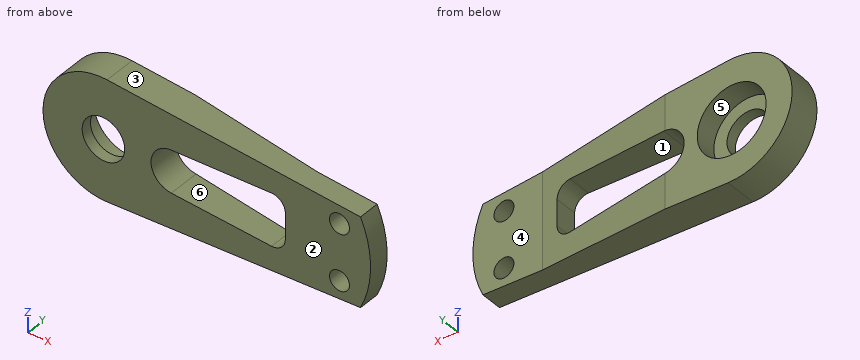
```python
from build123d import *

# Parameters (mm, degrees)
SKETCH1_R               = 1.9
SKETCH1_R_2             = 4.05
BOSS_EXTRUDE2_DEPTH     = 6
SKETCH2_R               = 6.55
CUT_EXTRUDE3_DEPTH      = 4
CUT_EXTRUDE2_DEPTH      = 21
CUT_EXTRUDE2_DEPTH_BACK = 16


with BuildPart() as part:
    # Sketch1 → Boss-Extrude2 (new body)
    with BuildSketch(Plane(origin=(0, 0, 0), x_dir=(1, 0, 0), z_dir=(0, 1, 0))):
        with BuildLine():
            Line((0.702058205, 11.478550182), (48.9, 8.530637776))
            ThreePointArc((48.9, 8.530637776), (50.810549507, 0), (48.9, -8.530637776))
            Line((48.9, -8.530637776), (0.702058205, -11.478550182))
            ThreePointArc((0.702058205, -11.478550182), (-11.5, 0), (0.702058205, 11.478550182))
        make_face()
        with Locations(Location((44.9, -5.35, 0), (0, 0, 270))):
            Circle(SKETCH1_R, mode=Mode.SUBTRACT)
        with Locations(Location((0, 0, 0), (0, 0, 270))):
            Circle(SKETCH1_R_2, mode=Mode.SUBTRACT)
        with Locations(Location((44.9, 5.35, 0), (0, 0, 270))):
            Circle(SKETCH1_R, mode=Mode.SUBTRACT)
        with BuildLine():
            Line((12.898162181, 4.044967428), (31.975408753, 4.996893474))
            ThreePointArc((31.975408753, 4.996893474), (33.823154358, 4.311281054), (34.6, 2.5))
            Line((34.6, 2.5), (34.6, -2.5))
            ThreePointArc((34.6, -2.5), (33.823154358, -4.311281054), (31.975408753, -4.996893474))
            Line((31.975408753, -4.996893474), (12.898162181, -4.044967428))
            ThreePointArc((12.898162181, -4.044967428), (9.05, 0), (12.898162181, 4.044967428))
        make_face(mode=Mode.SUBTRACT)
    extrude(amount=BOSS_EXTRUDE2_DEPTH)

    # Sketch2 → Cut-Extrude3 (cut)
    with BuildSketch(Plane(origin=(0, 6, 0), x_dir=(1, 0, 0), z_dir=(0, 1, 0))):
        with Locations(Location((0, 0, 0), (0, 0, 270))):
            Circle(SKETCH2_R)
    extrude(amount=-CUT_EXTRUDE3_DEPTH, mode=Mode.SUBTRACT)

    # Sketch3 → Cut-Extrude2 (cut, two sides: drawn at the far end of the back side and taken through both)
    with BuildSketch(Plane.XY.offset(-CUT_EXTRUDE2_DEPTH_BACK)):
        Polygon((50.810549507, 4), (37.603420494, 4), (12.707964704, 6), (50.810549507, 6), align=None)
    extrude(amount=CUT_EXTRUDE2_DEPTH + CUT_EXTRUDE2_DEPTH_BACK, mode=Mode.SUBTRACT)


solid = part.part
```
Can you work these out from the model? Positions are in its coordinate system, mm. Face numbers are marked on the shaded views. A direction names the side the tool comes from. Give positions to 0.01 mm unless a question says otherwise; leave off trailing zeros. Loops run counter-clockwise (first coordinate to the right, second up) from the corner with the lowest first, then second, coordinate; pieces in that order, holes last. Notation, with made-up numbers: M -15.75,-21.75 L 15.25,-21.75 A25 ccw 15.25,14.25 Z; hole C -23,75 d3. An arc over 180 degrees is marked long. One line per question, with ' | ' between items. Start each with the question number.
Q1. If we section it at C-C (y = 1.25): Please give me the cut outline in (x, z).
Q2. If we section it at A-A (z = 0): Please give me the cut outline in (x, y).
Q3. If we section it at D-D (x = 44.9): Please give me the cut outline in (y, z).
Q4. For pin 1 Ø2 at (y, z) = (2.5, 8) entering from +X; pin 2 Ø13 at (x, z) = (0, 0) entering from +Y; pin 3 Ø4 at (x, z) = (46, 2.5) entering from +Y, each with a flat end and sliding along its axis, tell me the tip position at first contact or that it passes through.
Q5. If we section it at B-B (x = 0): Please give me the cut outline in (y, z).
Q6. If we mould it in two halves opening along X, with no side actions, what happens to the marked faces 1, 2 and 3? For each: +X half, -X half, draft (parallel to the pull), parting line (faces both ways), or undercut.
Q7. If I drill on line 1 (Z direction, x = 44.9, y = 1.3); line 2 (X direction, y = 4.3, z = 0); line 3 (Y direction, x = -5, z = 1.25), over which ranges is the centre line in solid material (lowest first)? Write a range as from..to.
Q8. For the marked faces 4, 5 and 6, which set-ups out of +Z, -Z, +X, -X, +Y, -Y let a thin tool reach every point of the face, with its end or its side?
Computed:
1) outline: M 0.7,-11.48 L 48.9,-8.53 A20 ccw 48.9,8.53 L 0.7,11.48 A11.5 ccw long Z; hole C 0,0 d8.1; hole M 12.9,-4.04 L 31.98,-5 A2.5 ccw 34.6,-2.5 L 34.6,2.5 A2.5 ccw 31.98,5 L 12.9,4.04 A4.05 ccw Z; hole C 44.9,-5.35 d3.8; hole C 44.9,5.35 d3.8
2) outline: M -11.5,0 L -4.05,0 L -4.05,2 L -6.55,2 L -6.55,6 L -11.5,6 Z; M 4.05,0 L 9.05,0 L 9.05,6 L 6.55,6 L 6.55,2 L 4.05,2 Z; M 34.6,0 L 50.81,0 L 50.81,4 L 37.6,4 L 34.6,4.24 Z
3) outline: M 0,-8.78 L 4,-8.78 L 4,-7.25 L 0,-7.25 Z; M 0,-3.45 L 4,-3.45 L 4,3.45 L 0,3.45 Z; M 0,7.25 L 4,7.25 L 4,8.78 L 0,8.78 Z
4) pin 1: stops at x = 49.55 | pin 2: stops at y = 2 | pin 3: stops at y = 4
5) outline: M 0,-11.5 L 6,-11.5 L 6,-6.55 L 2,-6.55 L 2,-4.05 L 0,-4.05 Z; M 0,4.05 L 2,4.05 L 2,6.55 L 6,6.55 L 6,11.5 L 0,11.5 Z
6) face 1: undercut | face 2: draft | face 3: +X half
7) line 1: z = -8.78..-7.25, -3.45..3.45, 7.25..8.78 | line 2: x = -11.5..-6.55, 6.55..9.05 | line 3: y = 0..2
8) face 4: +Z, -Z, +X, +Y | face 5: +Y | face 6: +Y, -Y
